from build123d import *

# Parameters (mm, degrees)
CUT_EXTRUDE1_START       = -81.407
CUT_EXTRUDE1_OUTLINE_W   = 152.4
CUT_EXTRUDE1_OUTLINE_H   = 3.175
CUT_EXTRUDE1_DEPTH       = 84.582
CUT_EXTRUDE1_2_OUTLINE_R = 2.667
CUT_EXTRUDE1_2_DEPTH     = 3.175
CUT_EXTRUDE1_START_2     = -0.762
CUT_EXTRUDE1_3_OUTLINE_R = 2.667
CUT_EXTRUDE1_3_DEPTH     = 3.937
CUT_EXTRUDE1_START_3     = -78.232
CUT_EXTRUDE1_4_OUTLINE_R = 2.667
CUT_EXTRUDE1_4_DEPTH     = 0.762
CUT_EXTRUDE1_START_4     = 635
CUT_EXTRUDE1_5_DEPTH     = 152.4
CHAMFER1_SIZE            = 3.175
SKETCH2_W                = 38.1
SKETCH2_H                = 24.638
SKETCH2_R                = 2.667
CUT_EXTRUDE2_DEPTH       = 3.175
CHAMFER2_SIZE            = 3.175
CHAMFER3_SIZE            = 3.175


with BuildPart() as part:
    # Cut-Extrude1: read off the stored shape, not the designer's step
    # Cut-Extrude1 outline → Cut-Extrude1 (new body)
    with BuildSketch(Plane.XY.offset(CUT_EXTRUDE1_START)):
        with Locations((711.2, 1.5875)):
            Rectangle(CUT_EXTRUDE1_OUTLINE_W, CUT_EXTRUDE1_OUTLINE_H)
    extrude(amount=CUT_EXTRUDE1_DEPTH)

    # Cut-Extrude1 2 outline → Cut-Extrude1 2 (add)
    with BuildSketch(Plane.XY.offset(CUT_EXTRUDE1_START)):
        Polygon((635, 3.175), (787.4, 3.175), (787.4, 50.8), (784.225, 53.975), (635, 53.975), align=None)
        with Locations((641.35, 16.637)):
            Circle(CUT_EXTRUDE1_2_OUTLINE_R, mode=Mode.SUBTRACT)
        with Locations((654.05, 16.637)):
            Circle(CUT_EXTRUDE1_2_OUTLINE_R, mode=Mode.SUBTRACT)
        with Locations((666.75, 16.637)):
            Circle(CUT_EXTRUDE1_2_OUTLINE_R, mode=Mode.SUBTRACT)
        with Locations((679.45, 16.637)):
            Circle(CUT_EXTRUDE1_2_OUTLINE_R, mode=Mode.SUBTRACT)
        with Locations((692.15, 16.637)):
            Circle(CUT_EXTRUDE1_2_OUTLINE_R, mode=Mode.SUBTRACT)
        with Locations((704.85, 16.637)):
            Circle(CUT_EXTRUDE1_2_OUTLINE_R, mode=Mode.SUBTRACT)
        with Locations((717.55, 16.637)):
            Circle(CUT_EXTRUDE1_2_OUTLINE_R, mode=Mode.SUBTRACT)
        with Locations((730.25, 16.637)):
            Circle(CUT_EXTRUDE1_2_OUTLINE_R, mode=Mode.SUBTRACT)
        with Locations((742.95, 16.637)):
            Circle(CUT_EXTRUDE1_2_OUTLINE_R, mode=Mode.SUBTRACT)
        with Locations((755.65, 16.637)):
            Circle(CUT_EXTRUDE1_2_OUTLINE_R, mode=Mode.SUBTRACT)
        with Locations((768.35, 16.637)):
            Circle(CUT_EXTRUDE1_2_OUTLINE_R, mode=Mode.SUBTRACT)
        with Locations((781.05, 16.637)):
            Circle(CUT_EXTRUDE1_2_OUTLINE_R, mode=Mode.SUBTRACT)
        with Locations((768.35, 42.037)):
            Circle(CUT_EXTRUDE1_2_OUTLINE_R, mode=Mode.SUBTRACT)
        with Locations((781.05, 42.037)):
            Circle(CUT_EXTRUDE1_2_OUTLINE_R, mode=Mode.SUBTRACT)
        with Locations((641.35, 42.037)):
            Circle(CUT_EXTRUDE1_2_OUTLINE_R, mode=Mode.SUBTRACT)
        with Locations((654.05, 42.037)):
            Circle(CUT_EXTRUDE1_2_OUTLINE_R, mode=Mode.SUBTRACT)
        with Locations((666.75, 42.037)):
            Circle(CUT_EXTRUDE1_2_OUTLINE_R, mode=Mode.SUBTRACT)
        with Locations((679.45, 42.037)):
            Circle(CUT_EXTRUDE1_2_OUTLINE_R, mode=Mode.SUBTRACT)
        with Locations((692.15, 42.037)):
            Circle(CUT_EXTRUDE1_2_OUTLINE_R, mode=Mode.SUBTRACT)
        with Locations((704.85, 42.037)):
            Circle(CUT_EXTRUDE1_2_OUTLINE_R, mode=Mode.SUBTRACT)
        with Locations((717.55, 42.037)):
            Circle(CUT_EXTRUDE1_2_OUTLINE_R, mode=Mode.SUBTRACT)
        with Locations((730.25, 42.037)):
            Circle(CUT_EXTRUDE1_2_OUTLINE_R, mode=Mode.SUBTRACT)
        with Locations((742.95, 42.037)):
            Circle(CUT_EXTRUDE1_2_OUTLINE_R, mode=Mode.SUBTRACT)
        with Locations((755.65, 42.037)):
            Circle(CUT_EXTRUDE1_2_OUTLINE_R, mode=Mode.SUBTRACT)
    extrude(amount=CUT_EXTRUDE1_2_DEPTH)

    # Cut-Extrude1 3 outline → Cut-Extrude1 3 (add)
    with BuildSketch(Plane.XY.offset(CUT_EXTRUDE1_START_2)):
        Polygon((635, 34.925), (635, 3.175), (787.4, 3.175), (787.4, 31.75), (784.225, 34.925), align=None)
        with Locations((641.35, 16.637)):
            Circle(CUT_EXTRUDE1_3_OUTLINE_R, mode=Mode.SUBTRACT)
        with Locations((654.05, 16.637)):
            Circle(CUT_EXTRUDE1_3_OUTLINE_R, mode=Mode.SUBTRACT)
        with Locations((666.75, 16.637)):
            Circle(CUT_EXTRUDE1_3_OUTLINE_R, mode=Mode.SUBTRACT)
        with Locations((679.45, 16.637)):
            Circle(CUT_EXTRUDE1_3_OUTLINE_R, mode=Mode.SUBTRACT)
        with Locations((692.15, 16.637)):
            Circle(CUT_EXTRUDE1_3_OUTLINE_R, mode=Mode.SUBTRACT)
        with Locations((704.85, 16.637)):
            Circle(CUT_EXTRUDE1_3_OUTLINE_R, mode=Mode.SUBTRACT)
        with Locations((717.55, 16.637)):
            Circle(CUT_EXTRUDE1_3_OUTLINE_R, mode=Mode.SUBTRACT)
        with Locations((730.25, 16.637)):
            Circle(CUT_EXTRUDE1_3_OUTLINE_R, mode=Mode.SUBTRACT)
        with Locations((742.95, 16.637)):
            Circle(CUT_EXTRUDE1_3_OUTLINE_R, mode=Mode.SUBTRACT)
        with Locations((755.65, 16.637)):
            Circle(CUT_EXTRUDE1_3_OUTLINE_R, mode=Mode.SUBTRACT)
        with Locations((768.35, 16.637)):
            Circle(CUT_EXTRUDE1_3_OUTLINE_R, mode=Mode.SUBTRACT)
        with Locations((781.05, 16.637)):
            Circle(CUT_EXTRUDE1_3_OUTLINE_R, mode=Mode.SUBTRACT)
    extrude(amount=CUT_EXTRUDE1_3_DEPTH)

    # Cut-Extrude1 4 outline → Cut-Extrude1 4 (add)
    with BuildSketch(Plane.XY.offset(CUT_EXTRUDE1_START_3)):
        Polygon((635, 34.925), (635, 3.175), (787.4, 3.175), (787.4, 31.75), (784.225, 34.925), align=None)
        with Locations((641.35, 16.637)):
            Circle(CUT_EXTRUDE1_4_OUTLINE_R, mode=Mode.SUBTRACT)
        with Locations((654.05, 16.637)):
            Circle(CUT_EXTRUDE1_4_OUTLINE_R, mode=Mode.SUBTRACT)
        with Locations((666.75, 16.637)):
            Circle(CUT_EXTRUDE1_4_OUTLINE_R, mode=Mode.SUBTRACT)
        with Locations((679.45, 16.637)):
            Circle(CUT_EXTRUDE1_4_OUTLINE_R, mode=Mode.SUBTRACT)
        with Locations((692.15, 16.637)):
            Circle(CUT_EXTRUDE1_4_OUTLINE_R, mode=Mode.SUBTRACT)
        with Locations((704.85, 16.637)):
            Circle(CUT_EXTRUDE1_4_OUTLINE_R, mode=Mode.SUBTRACT)
        with Locations((717.55, 16.637)):
            Circle(CUT_EXTRUDE1_4_OUTLINE_R, mode=Mode.SUBTRACT)
        with Locations((730.25, 16.637)):
            Circle(CUT_EXTRUDE1_4_OUTLINE_R, mode=Mode.SUBTRACT)
        with Locations((742.95, 16.637)):
            Circle(CUT_EXTRUDE1_4_OUTLINE_R, mode=Mode.SUBTRACT)
        with Locations((755.65, 16.637)):
            Circle(CUT_EXTRUDE1_4_OUTLINE_R, mode=Mode.SUBTRACT)
        with Locations((768.35, 16.637)):
            Circle(CUT_EXTRUDE1_4_OUTLINE_R, mode=Mode.SUBTRACT)
        with Locations((781.05, 16.637)):
            Circle(CUT_EXTRUDE1_4_OUTLINE_R, mode=Mode.SUBTRACT)
    extrude(amount=CUT_EXTRUDE1_4_DEPTH)

    # Cut-Extrude1 5 outline → Cut-Extrude1 5 (cut)
    with BuildSketch(Plane.YZ.offset(CUT_EXTRUDE1_START_4)):
        with BuildLine():
            Line((0, -81.407), (3.937, -81.407))
            ThreePointArc((3.937, -81.407), (1.153120602, -80.253879398), (0, -77.47))
            Line((0, -77.47), (0, -81.407))
        make_face()
        with BuildLine():
            Line((34.925, -0.762), (34.925, 0))
            Line((34.925, 0), (3.937, 0))
            ThreePointArc((3.937, 0), (3.398184633, -0.223184633), (3.175, -0.762))
            Line((3.175, -0.762), (34.925, -0.762))
        make_face()
        with BuildLine():
            Line((0, 3.175), (0, -0.762))
            ThreePointArc((0, -0.762), (1.153120602, 2.021879398), (3.937, 3.175))
            Line((3.937, 3.175), (0, 3.175))
        make_face()
        with BuildLine():
            ThreePointArc((3.175, -77.47), (3.398184633, -78.008815367), (3.937, -78.232))
            Line((3.937, -78.232), (34.925, -78.232))
            Line((34.925, -78.232), (34.925, -77.47))
            Line((34.925, -77.47), (3.175, -77.47))
        make_face()
    extrude(amount=CUT_EXTRUDE1_5_DEPTH, mode=Mode.SUBTRACT)

    # Chamfer1
    chamfer1_edges = [part.edges().sort_by_distance(p)[0] for p in [
        (635, 34.925, 1.5875),
        (635, 53.975, -79.8195),
    ]]
    chamfer(chamfer1_edges, length=CHAMFER1_SIZE)

    # Sketch2 → Cut-Extrude2 (cut)
    with BuildSketch(Plane(origin=(0, 0, -81.407), x_dir=(-1, 0, 0), z_dir=(0, 0, -1))):
        with Locations((-692.15, 41.656)):
            Rectangle(SKETCH2_W, SKETCH2_H)
        with Locations((-704.85, 42.037)):
            Circle(SKETCH2_R, mode=Mode.SUBTRACT)
        with Locations((-692.15, 42.037)):
            Circle(SKETCH2_R, mode=Mode.SUBTRACT)
        with Locations((-679.45, 42.037)):
            Circle(SKETCH2_R, mode=Mode.SUBTRACT)
    extrude(amount=-CUT_EXTRUDE2_DEPTH, mode=Mode.SUBTRACT)

    # Chamfer2
    chamfer2_edges = [part.edges().sort_by_distance(p)[0] for p in [
        (711.2, 53.975, -79.8195),
        (673.1, 53.975, -79.8195),
    ]]
    chamfer(chamfer2_edges, length=CHAMFER2_SIZE)

    # Chamfer3
    chamfer3_edges = [part.edges().sort_by_distance(p)[0] for p in [
        (711.2, 29.337, -79.8195),
        (673.1, 29.337, -79.8195),
    ]]
    chamfer(chamfer3_edges, length=CHAMFER3_SIZE)


solid = part.part
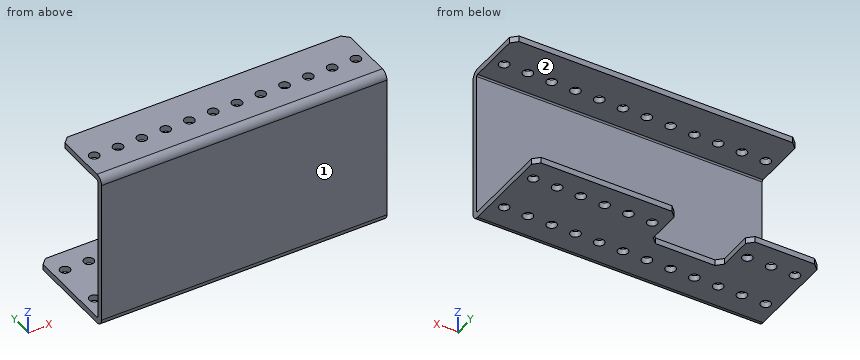
Design review of the part built by this model. Coordinates are the model's own, in mm. Face numbers are marked on the shaded views. A direction names the side the tool comes from. Coordinates: 2 decimals unless noted, no trailing zeros. Write each loop counter-clockwise with the first axis right and the second up, starting at its lowest first coordinate (ties: lowest second). Pieces come first, ordered by that corner, then holes. Notation, with made-up numbers: (-37.5, -8.5) - (12.5, -8.5) arc R13 ccw to (12.5, 6.5) - close; hole circle Ø2 at (-22, -4.5). An arc over 180 degrees is marked (long way). One line per item, written item: value.
1) Add section C-C (y = 27.5). State the section outline as (x, z) points (3 decimals), plus the area to 3 significant figures.
Answer sheet:
outline: (635, -81.407) - (787.4, -81.407) - (787.4, -78.232) - (635, -78.232) - close; (635, 0) - (787.4, 0) - (787.4, 3.175) - (635, 3.175) - close
area: 968 mm2
2) Add section D-D (z = -41). State the section outline as (x, y) points (3 decimals).
Answer sheet:
outline: (635, 0) - (787.4, 0) - (787.4, 3.175) - (635, 3.175) - close
3) Insertion check: pin 1 (5 mm diameter, centred on x = 730.25, y = 16.637, fed in from -Z); pin 2 (12 mm diameter, centred on x = 709, z = -19, fed in from +Y) (3 decimals); pin 3 (1 mm diameter, centred on x = 694.5, z = -80, fed in from +Y); pin 4 (6 mm diameter, centred on x = 781.05, y = 42.037, fed in from +Z). Each pin has a flat end and moves straight along its axis. Give the tip position at first contact, or say it passes through.
Answer sheet:
pin 1: passes through
pin 2: stops at y = 3.175
pin 3: stops at y = 29.34
pin 4: stops at z = -78.23
4) To check wall thickness, follow probe 1 along Z at (x, y) = (662, 20.5) (3 decimals); probe 2 along Y at (x, z) = (730.25, -80.65) (3 decimals); probe 3 along Y at (x, z) = (730.25, -80.45) (3 decimals). State the ranges of each line that lie inside material, in increasing order.
Answer sheet:
probe 1: z = -81.407 to -78.232, 0 to 3.175
probe 2: y = 1.616 to 13.97, 19.304 to 39.37, 44.704 to 53.975
probe 3: y = 1.364 to 13.97, 19.304 to 39.37, 44.704 to 53.975
5) Add section B-B (x = 692.15). State the section outline as (y, z) points (3 decimals), plus the area to 3 significant figures.
Answer sheet:
outline: (0, -77.47) arc R3.937 ccw to (3.937, -81.407) - (13.97, -81.407) - (13.97, -78.232) - (3.937, -78.232) arc R0.762 cw to (3.175, -77.47) - (3.175, -0.762) arc R0.762 cw to (3.937, 0) - (13.97, 0) - (13.97, 3.175) - (3.937, 3.175) arc R3.937 ccw to (0, -0.762) - close; (19.304, -81.407) - (29.337, -81.407) - (29.337, -78.232) - (19.304, -78.232) - close; (19.304, 0) - (34.925, 0) - (34.925, 3.175) - (19.304, 3.175) - close
area: 412 mm2
6) For the marked faces 1 and 2, list the 3-axis set-ups (+Z, -Z, +X, -X, +Y, -Y) from which the entire face can be reached by the end or side of a thin tool; tool diameter is ignored.
Answer sheet:
face 1: +Z, -Z, +X, -X, -Y
face 2: +X, -X, +Y
7) Add section A-A (x = 666.75). State the section outline as (y, z) points (3 decimals), plus the area to 3 significant figures.
Answer sheet:
outline: (0, -77.47) arc R3.937 ccw to (3.937, -81.407) - (13.97, -81.407) - (13.97, -78.232) - (3.937, -78.232) arc R0.762 cw to (3.175, -77.47) - (3.175, -0.762) arc R0.762 cw to (3.937, 0) - (13.97, 0) - (13.97, 3.175) - (3.937, 3.175) arc R3.937 ccw to (0, -0.762) - close; (19.304, -81.407) - (39.37, -81.407) - (39.37, -78.232) - (19.304, -78.232) - close; (19.304, 0) - (34.925, 0) - (34.925, 3.175) - (19.304, 3.175) - close; (44.704, -81.407) - (53.975, -81.407) - (53.975, -78.232) - (44.704, -78.232) - close
area: 473 mm2
